Here's how the part is built. I have some questions about the finished solid (model axes, mm). A direction names the side the tool comes from. Coordinates: 2 decimals unless noted, no trailing zeros. Write each loop counter-clockwise with the first axis right and the second up, starting at its lowest first coordinate (ties: lowest second). Pieces come first, ordered by that corner, then holes. Notation, with made-up numbers: (88.25, -12.5) -> (133.25, -12.5) arc R27 ccw to (133.25, 15.5) -> close; hole circle Ø7 at (83.5, -4). An arc over 180 degrees is marked (long way). Put each result on its own line as item: value. Start each with the question number.
Item 1: For pin 1 (4 mm diameter, centred on y = -7.5, z = 64, fed in from -X) (3 decimals); pin 2 (2 mm diameter, centred on x = 34.5, z = 11.5, fed in from +Y); pin 3 (10 mm diameter, centred on x = -0.5, z = 16.5, fed in from -Y), each with a flat end and sliding along its axis, tell me the tip position at first contact or that it passes through.
Item 2: On a 3-axis mill with a long thin cutter (end or side, diameter ignored), from which of +Z, -Z, +X, -X, +Y, -Y can I reach the whole of each face in a straight line? I mean faces 1 (the face through (41.275, -14, 4)), 2 (the face through (36, -25.4, 39)), 3 (the face through (36, 25.4, 39)), 4 (the face through (60.325, 0, 64)). Say none if no direction works.
Item 3: I want a section at A-A, the plane x = 84. List the corners of the cut face in (y, z) for me (3 decimals).
Item 4: I want a section at B-B, the plane y = -48.5. List the corners of the cut face in (x, z) for me (3 decimals), then the cut area to 3 significant figures.
Item 5: I need wall thicknesses on line 1 (Y direction, x = 2.5, z = 25.5); line 2 (X direction, y = -64.5, z = 3) (3 decimals); line 3 (Z direction, x = 34, y = -59) (3 decimals). Which ranges of each line are inside material? Lowest first, please. Write a range as [from, to].
from build123d import *

# Parameters (mm, degrees)
F0_W     = 25.4
F0_H     = 19.05
F1_DEPTH = 25.4
F2_DEPTH = 12.7
F3_DEPTH = 63.5


# Not quite as in the source:
# - a feature of the source that left no trace in its solid (it failed there, or was rolled back) is left out


with BuildPart() as f1:
    # F0 (on Front) → F1 (new body, symmetric)
    with BuildSketch(Plane.XZ):
        with BuildLine():
            add(Edge.make_bspline(
                [(-41.275, 9.525), (-39.3446406739, 28.5086459931), (-0.7471661584, 60.2765032574), (55.5187541124, 61.8870838083)],
                knots=[0, 0, 0, 0, 110.4404580892, 110.4404580892, 110.4404580892, 110.4404580892], degree=3))
            Line((-41.275, 9.525), (22.225, 9.525))
            Line((22.225, 9.525), (22.225, 27.0002))
            ThreePointArc((22.225, 27.0002), (31.8841447045, 51.1122754227), (55.5187541124, 61.8870838083))
        make_face()
        with BuildLine():
            Line((22.225, 9.525), (41.275, 9.525))
            Line((41.275, 9.525), (41.275, 27.0002))
            ThreePointArc((41.275, 27.0002), (45.9246798487, 38.2255201513), (57.15, 42.8752))
            Line((57.15, 42.8752), (60.325, 42.8752))
            Line((60.325, 42.8752), (60.325, 61.9252))
            Line((60.325, 61.9252), (57.15, 61.9252))
            add(Edge.make_bspline(
                [(55.5187541124, 61.8870838083), (56.0608682355, 61.9026015224), (56.6046225289, 61.915319722), (57.15, 61.9252)],
                knots=[110.4404580892, 110.4404580892, 110.4404580892, 110.4404580892, 111.5045361635, 111.5045361635, 111.5045361635, 111.5045361635], degree=3))
            ThreePointArc((55.5187541124, 61.8870838083), (31.8841447045, 51.1122754227), (22.225, 27.0002))
            Line((22.225, 27.0002), (22.225, 9.525))
        make_face()
        with Locations((73.025, 52.4002)):
            Rectangle(F0_W, F0_H)
        Polygon((60.325, 66.675), (60.325, 61.9252), (85.725, 61.9252), (85.725, 42.8752), (60.325, 42.8752), (60.325, 38.1), (111.125, 38.1), (111.125, 66.675), align=None)
    extrude(amount=F1_DEPTH, both=True)

    # F0 (on Front) → F2 (join, symmetric)
    with BuildSketch(Plane.XZ):
        Polygon((-41.275, 9.525), (-41.275, -9.525), (41.275, -9.525), (41.275, 9.525), (22.225, 9.525), align=None)
        with BuildLine():
            add(Edge.make_bspline(
                [(-41.275, 9.525), (-39.3446406739, 28.5086459931), (-0.7471661584, 60.2765032574), (55.5187541124, 61.8870838083)],
                knots=[0, 0, 0, 0, 110.4404580892, 110.4404580892, 110.4404580892, 110.4404580892], degree=3))
            Line((-41.275, 9.525), (22.225, 9.525))
            Line((22.225, 9.525), (22.225, 27.0002))
            ThreePointArc((22.225, 27.0002), (31.8841447045, 51.1122754227), (55.5187541124, 61.8870838083))
        make_face()
        with BuildLine():
            Line((22.225, 9.525), (41.275, 9.525))
            Line((41.275, 9.525), (41.275, 27.0002))
            ThreePointArc((41.275, 27.0002), (45.9246798487, 38.2255201513), (57.15, 42.8752))
            Line((57.15, 42.8752), (60.325, 42.8752))
            Line((60.325, 42.8752), (60.325, 61.9252))
            Line((60.325, 61.9252), (57.15, 61.9252))
            add(Edge.make_bspline(
                [(55.5187541124, 61.8870838083), (56.0608682355, 61.9026015224), (56.6046225289, 61.915319722), (57.15, 61.9252)],
                knots=[110.4404580892, 110.4404580892, 110.4404580892, 110.4404580892, 111.5045361635, 111.5045361635, 111.5045361635, 111.5045361635], degree=3))
            ThreePointArc((55.5187541124, 61.8870838083), (31.8841447045, 51.1122754227), (22.225, 27.0002))
            Line((22.225, 27.0002), (22.225, 9.525))
        make_face()
        with Locations((73.025, 52.4002)):
            Rectangle(F0_W, F0_H)
        Polygon((60.325, 66.675), (60.325, 61.9252), (85.725, 61.9252), (85.725, 42.8752), (60.325, 42.8752), (60.325, 38.1), (111.125, 38.1), (111.125, 66.675), align=None)
    extrude(amount=F2_DEPTH, both=True)

    # F3 (add, symmetric): a face of the model
    f3_faces = [f1.faces().sort_by_distance(p)[0] for p in [
        (0, -12.7, 0),
    ]]
    extrude(f3_faces, amount=F3_DEPTH, both=True)


solid = f1.part
Calculated:
1. pin 1: stops at x = 60.325
1. pin 2: stops at y = 25.4
1. pin 3: stops at y = -25.4
2. face 1: -Z, +X, +Y, -Y
2. face 2: +Z, +X, -X, -Y
2. face 3: +Z, +X, -X, +Y
2. face 4: +Z, -X, +Y, -Y
3. outline: (-25.4, 38.1) -> (25.4, 38.1) -> (25.4, 66.675) -> (-25.4, 66.675) -> close
4. outline: (-41.275, -9.525) -> (41.275, -9.525) -> (41.275, 9.525) -> (-41.275, 9.525) -> close
4. area: 1,570 mm2
5. line 1: y = [-25.4, 25.4]
5. line 2: x = [-41.275, 41.275]
5. line 3: z = [-9.525, 9.525]
